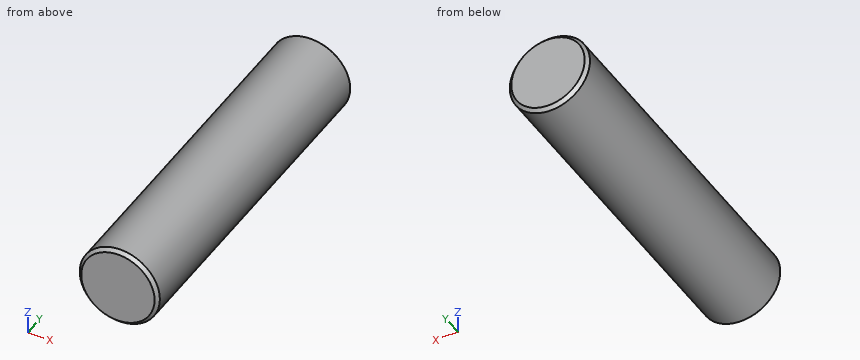
```python
from build123d import *

# Parameters (mm, degrees)
SKETCH1_R           = 2.95
BOSS_EXTRUDE1_DEPTH = 25.6
CHAMFER3_SIZE       = 0.25
CHAMFER4_SIZE       = 0.25


with BuildPart() as part:
    # Sketch1 → Boss-Extrude1 (new body)
    with BuildSketch(Plane(origin=(0, 0, 0), x_dir=(1, 0, 0), z_dir=(0, 1, 0))):
        Circle(SKETCH1_R)
    extrude(amount=-BOSS_EXTRUDE1_DEPTH)

    # Chamfer3
    chamfer3_edges = [part.edges().sort_by_distance(p)[0] for p in [
        (-2.95, -25.6, 0),
    ]]
    chamfer(chamfer3_edges, length=CHAMFER3_SIZE)

    # Chamfer4
    chamfer4_edges = [part.edges().sort_by_distance(p)[0] for p in [
        (-2.95, 0, 0),
    ]]
    chamfer(chamfer4_edges, length=CHAMFER4_SIZE)


solid = part.part
```
Part model, mm, in its own coordinate system. Round coordinates to 2 decimals unless told otherwise and drop trailing zeros. Write each loop counter-clockwise with the first axis right and the second up, starting at its lowest first coordinate (ties: lowest second). Pieces come first, ordered by that corner, then holes. Notation, with made-up numbers: M -6.5,74 L 1.5,74 A31 cw 1.5,110 Z; hole C 73,-33.75 d1. An arc over 180 degrees is marked long. Answer as CSV lines item,"result". Start each with the question number.
1) Drop a flat-ended pin along its axis: pin 1 (1 mm diameter, centred on x = -1.5, y = -4.5, fed in from +Z). Give the stop position or say it passes through.
2) Drill centre lines: L1, parallel to X at y = -5.5, z = -1.2; L2, parallel to Z at x = -0.45, y = -19.25; L3, parallel to X at y = -2, z = -1.3. Where is each one in solid material? Low to high.
3) Band-saw the part on A-A (y = -3). List the corners of the cut face in (x, z), then the cut area to 3 significant figures.
Worked out:
1,pin 1,"z = 2.78"
2,L1,"-2.69 to 2.69"
2,L2,"-2.92 to 2.92"
2,L3,"-2.65 to 2.65"
3,outline,"C 0,0 d5.9"
3,area,"27.3 mm²"
